from build123d import *

# Parameters (mm, degrees)
BOSS_EXTRUDE1_DEPTH     = 30
BOSS_EXTRUDE2_DEPTH     = 12
BOSS_EXTRUDE3_DEPTH     = 8
CUT_EXTRUDE1_DEPTH      = 72.589105316
CUT_EXTRUDE1_DEPTH_BACK = 72.589105316


with BuildPart() as part:
    # Sketch2 → Boss-Extrude1 (new body)
    with BuildSketch(Plane.XY):
        Polygon((0, 0), (56, 0), (56, 8), (32, 8), (32, 12), (0, 12), align=None)
    extrude(amount=BOSS_EXTRUDE1_DEPTH)

    # Sketch3 → Boss-Extrude2 (add)
    with BuildSketch(Plane.XY):
        with BuildLine():
            Line((32, 8), (32, 21))
            ThreePointArc((32, 21), (44, 33), (56, 21))
            Line((56, 21), (56, 8))
            Line((56, 8), (32, 8))
        make_face()
        with BuildLine():
            Line((50, 21), (50, 16))
            ThreePointArc((50, 16), (44, 10), (38, 16))
            Line((38, 16), (38, 21))
            ThreePointArc((38, 21), (44, 27), (50, 21))
        make_face(mode=Mode.SUBTRACT)
    extrude(amount=BOSS_EXTRUDE2_DEPTH)

    # Sketch4 → Boss-Extrude3 (add)
    with BuildSketch(Plane.XY):
        with BuildLine():
            Line((0, 20), (0, 12))
            Line((0, 12), (32, 12))
            Line((32, 12), (32, 21))
            ThreePointArc((32, 21), (34.251977355, 27.998289399), (40.162675751, 32.369913923))
            Line((40.162675751, 32.369913923), (0, 20))
        make_face()
    extrude(amount=BOSS_EXTRUDE3_DEPTH)

    # Sketch5 → Cut-Extrude1 (cut, two sides: drawn at the far end of the back side and taken through both)
    with BuildSketch(Plane.ZY.offset(-CUT_EXTRUDE1_DEPTH_BACK)):
        Polygon((9, 0), (21, 0), (23.886751346, 5), (6.113248654, 5), align=None)
    extrude(amount=CUT_EXTRUDE1_DEPTH + CUT_EXTRUDE1_DEPTH_BACK, mode=Mode.SUBTRACT)


solid = part.part
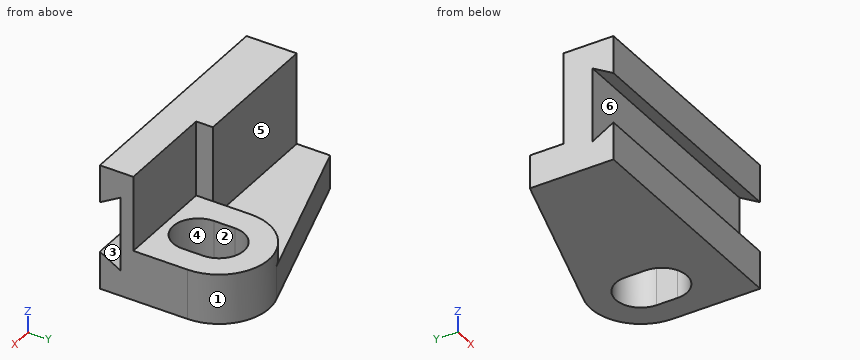
Verification items for the finished model (mm, model axes). Face numbers are marked on the shaded views. A direction names the side the tool comes from. Give positions to 0.01 mm unless a question says otherwise; leave off trailing zeros. Loops run counter-clockwise (first coordinate to the right, second up) from the corner with the lowest first, then second, coordinate; pieces in that order, holes last.
1) Draft check along X on the marked faces 1, 2 and 3. Enter one of: pulls with the +X half, pulls with the -X half, needs draft (parallel to the pull), parting line crosses it, or undercut.
2) Sectioned sample at D-D, the plane y = 4. Enter the section's corners in (x, z), then the cut area to 3 significant figures.
3) Sectioned sample at B-B, the plane y = 24. Enter the section's corners in (x, z), then the cut area to 3 significant figures.
4) Sectioned sample at A-A, the plane x = 44. Enter the section's corners in (y, z), then the cut area to 3 significant figures.
5) Sectioned sample at C-C, the plane x = 28.5. Enter the section's corners in (y, z), then the cut area to 3 significant figures.
6) Thickness scan on line 1 along Y through (x, z) = (4.5, 19.5); line 2 along Z through (x, y) = (27.5, 3); line 3 along Y through (x, z) = (47, 24.5). Record the ranges inside material, lowest first.
7) Set-up check for the marked faces 4, 5 and 6: record each of +Z, -Z, +X, -X, +Y, -Y from which the full face is reachable in a straight line by a thin tool's end or side.
8) Depth check by flat-ended pin: pin 1 Ø4.5 at (y, z) = (14.5, 10.5) entering from -X; pin 2 Ø14.5 at (x, z) = (38, 22) entering from +Y; pin 3 Ø3 at (x, z) = (42, 13) entering from -Y. Enter the tip coordinate at first touch or a pass-through.
Answers:
1. face 1: parting line crosses it
1. face 2: undercut
1. face 3: needs draft
2. outline: (0, 0) - (56, 0) - (56, 6.69) - (0, 6.69) - close; (0, 23.31) - (56, 23.31) - (56, 30) - (0, 30) - close
2. area: 749 mm2
3. outline: (12.99, 0) - (38.8, 0) - (38.8, 12) - (32.38, 12) - (32.38, 8) - (12.99, 8) - close; (49.2, 0) - (55.62, 0) - (55.62, 12) - (49.2, 12) - close
3. area: 309 mm2
4. outline: (0, 0) - (10, 0) - (10, 12) - (8, 12) - (8, 30) - (0, 30) - (0, 21) - (5, 23.89) - (5, 6.11) - (0, 9) - close; (27, 0) - (33, 0) - (33, 12) - (27, 12) - close
4. area: 262 mm2
5. outline: (0, 0) - (28.78, 0) - (28.78, 8) - (12, 8) - (12, 30) - (0, 30) - (0, 21) - (5, 23.89) - (5, 6.11) - (0, 9) - close
5. area: 420 mm2
6. line 1: y = 5 to 12
6. line 2: z = 0 to 7.27, 22.73 to 30
6. line 3: y = 0 to 8
7. face 4: +Z, -Z
7. face 5: +Z, -X, +Y
7. face 6: +X, -X
8. pin 1: stops at x = 32
8. pin 2: stops at y = 12
8. pin 3: stops at y = 5
